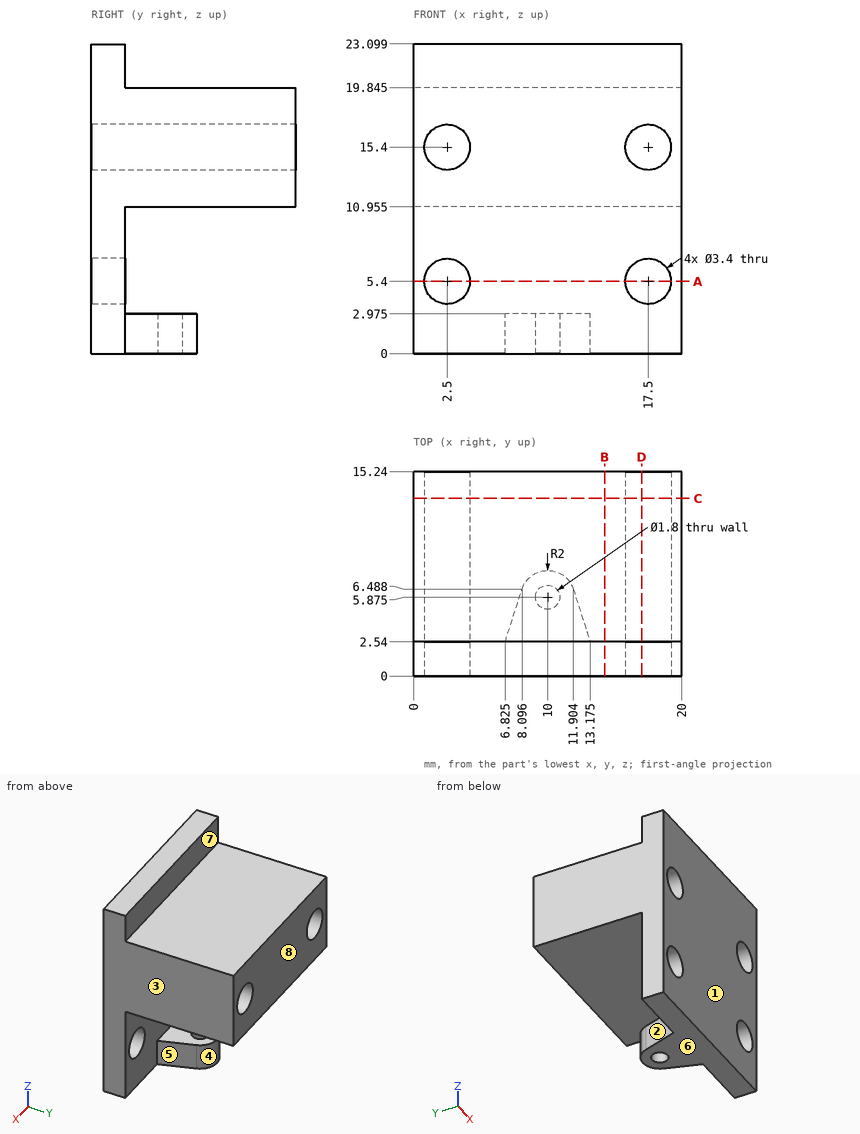
Geometry: see drawing. Coordinates: mm, zero at the bounding-box minimum. A direction names the side the tool comes from. Give positions to 0.01 mm unless a question says otherwise; leave off trailing zeros. Write each loop counter-clockwise with the first axis right and the second up, starting at its lowest first coordinate (ties: lowest second). Pieces come first, ordered by that corner, then holes. Notation, with made-up numbers: M 65,-36.5 L 76,-36.5 A22 ccw 76,0.5 Z; hole C 29.25,52 d9. An arc over 180 degrees is marked long. Answer as a JSON object with one key per item and string values.
Q1. Access query for the marked faces 4, 5, 6, 7 and 8. Directions: +Z, -Z, +X, -X, +Y, -Y. A direction counts if a zero-diameter tool reaches every point of the face in a straight line with its end or side. Return the directions, or none.
Geometry check:
{"face 4": "-Z, +Y", "face 5": "-Z, +X, +Y", "face 6": "-Z, +X, -X, +Y, -Y", "face 7": "+Z, +X, -X, +Y", "face 8": "+Z, -Z, +X, -X, +Y"}
Q2. Mould query, pull axis X, two halves, no side actions, for the marked faces 1, 2 and 3. Classes: +X half, -X half, draft (parallel to the pull), parting line (faces both ways), or undercut.
Geometry check:
{"face 1": "draft", "face 2": "-X half", "face 3": "+X half"}
Q3. Cut plane C-C, the plane y = 13.25. Return the cut outline in (x, z) (1 decimal).
Geometry check:
{"outline": "M 0,11 L 20,11 L 20,19.8 L 0,19.8 Z; hole C 2.5,15.4 d3.4; hole C 17.5,15.4 d3.4"}
Q4. Cut plane A-A, the plane z = 5.4. Return the cut outline in (x, y).
Geometry check:
{"outline": "M 0,0 L 0.8,0 L 0.8,2.54 L 0,2.54 Z; M 4.2,0 L 15.8,0 L 15.8,2.54 L 4.2,2.54 Z; M 19.2,0 L 20,0 L 20,2.54 L 19.2,2.54 Z"}
Q5. Cut plane B-B, the plane x = 14.25. Return the cut outline in (y, z) (1 decimal), then the cut area to 3 significant figures.
Geometry check:
{"outline": "M 0,0 L 2.5,0 L 2.5,11 L 15.2,11 L 15.2,19.8 L 2.5,19.8 L 2.5,23.1 L 0,23.1 Z", "area": "172 mm^2"}
Q6. Ray query, line 1 along Z through (x, y) = (17.5, 10.25) (1 decimal); line 2 along Y through (x, z) = (9.25, 20.25); line 3 along Z through (x, y) = (18, 7.5) (1 decimal). Return the intervals inside material, ascending.
Geometry check:
{"line 1": "z = 11 to 13.7, 17.1 to 19.8", "line 2": "y = 0 to 2.54", "line 3": "z = 11 to 13.8, 17 to 19.8"}
Q7. Contact query for flat-ended pins moving along their axis: P1, Ø1, axis at x = 14, z = 21.5, coming from the +Y side; P2, Ø1, axis at x = 10.5, y = 7, coming from the +Z side (3 decimals); P3, Ø1.5, axis at x = 16.5, y = 7.5, coming from the -Z side (3 decimals). Output: stop coordinate, or through.
Geometry check:
{"P1": "stops at y = 2.54", "P2": "stops at z = 19.845", "P3": "stops at z = 10.955"}
Q8. Cut plane D-D, the plane x = 17. Return the cut outline in (y, z) (1 decimal), then the cut area to 3 significant figures.
Geometry check:
{"outline": "M 0,0 L 2.5,0 L 2.5,3.8 L 0,3.8 Z; M 0,7 L 2.5,7 L 2.5,11 L 15.2,11 L 15.2,13.8 L 0,13.8 Z; M 0,17 L 15.2,17 L 15.2,19.8 L 2.5,19.8 L 2.5,23.1 L 0,23.1 Z", "area": "114 mm^2"}
